The drawing under review shows one solid part. Ordinate dimensions are in mm from its lowest x, y, z. A direction names the side the tool comes from. Coordinates: 2 decimals unless noted, no trailing zeros. Order: outer loops, then holes, each group sorted by start corner. A loop starts at its lowest first (then second) coordinate and runs counter-clockwise, first axis right, second up. Notation, with made-up numbers: M 52.5,50.5 L 103.5,50.5 A15 ccw 103.5,77.5 Z; hole C 59,-10 d1. An arc over 180 degrees is marked long. Answer as a JSON object with one key per item and string values.
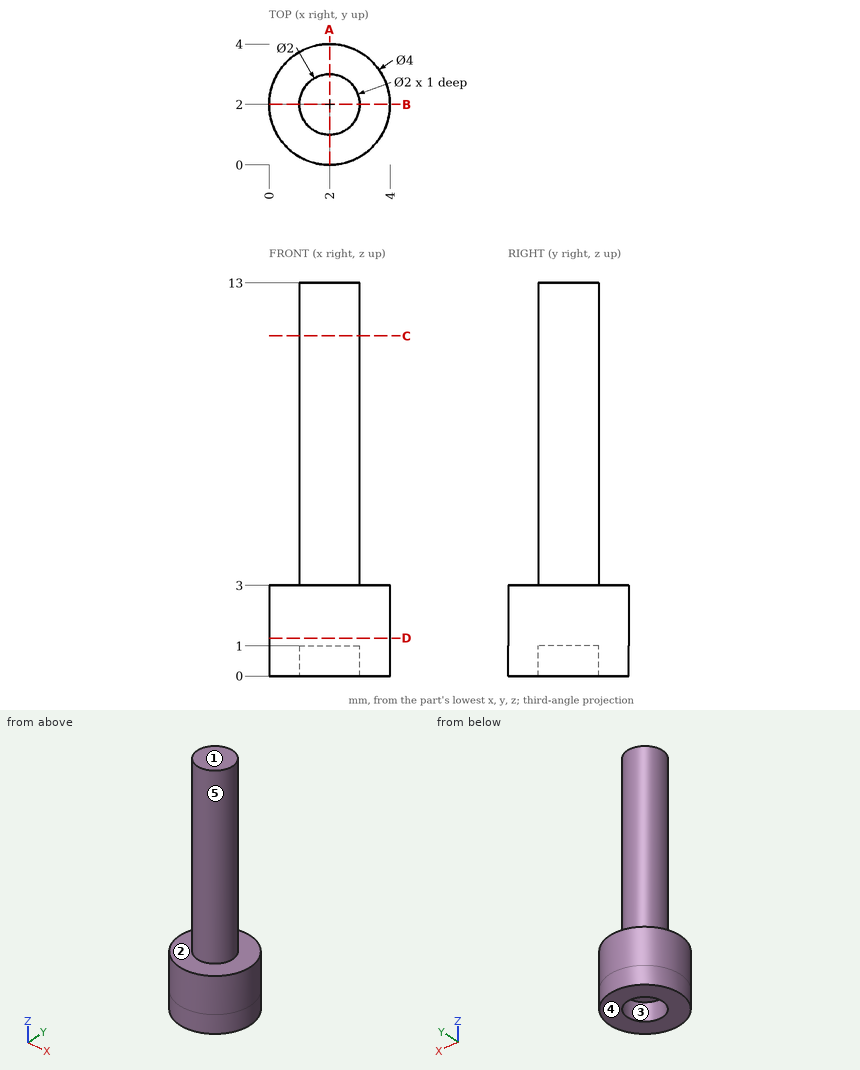
1) Add section D-D (z = 1.25). State the section outline as (x, y) points, and give its area (3 significant figures).
Taken from the geometry:
{"outline": "C 2,2 d4", "area": "12.6 mm2"}
2) To check wall thickness, follow L1, parallel to Y at x = 2, z = 0.2; L2, parallel to Z at x = 2.8, y = 1.05; L3, parallel to Z at x = 2.15, y = 1.85. State the ranges of each line that lie inside material, in increasing order.
Taken from the geometry:
{"L1": "y = 0 to 1, 3 to 4", "L2": "z = 0 to 3", "L3": "z = 1 to 13"}
3) Add section A-A (x = 2). State the section outline as (y, z) points.
Taken from the geometry:
{"outline": "M 0,0 L 1,0 L 1,1 L 3,1 L 3,0 L 4,0 L 4,3 L 3,3 L 3,13 L 1,13 L 1,3 L 0,3 Z"}
4) Add section C-C (z = 11.25). State the section outline as (x, y) points, and give its area (3 significant figures).
Taken from the geometry:
{"outline": "C 2,2 d2", "area": "3.14 mm2"}
5) Insertion check: pin 1 Ø2 at (y, z) = (1.5, 7) entering from +X; pin 2 Ø1.6 at (x, y) = (2, 2) entering from -Z. Each pin has a flat end and moves straight along its axis. Give the tip position at first contact, or say it passes through.
Taken from the geometry:
{"pin 1": "stops at x = 3", "pin 2": "stops at z = 1"}
6) Tool access review of the marked faces 1 and 2: name each direction out of +Z, -Z, +X, -X, +Y, -Y from which nothing blocks a thin tool from reaching the whole face with its end or side.
Taken from the geometry:
{"face 1": "+Z, +X, -X, +Y, -Y", "face 2": "+Z"}
7) Mouldability with a two-part tool opening along Y and no side actions: class the marked faces 3, 4 and 5 as released by +Y, released by -Y, zero draft, split by the parting line, or undercut.
Taken from the geometry:
{"face 3": "undercut", "face 4": "zero draft", "face 5": "split by the parting line"}
